Autodesk Inventor part; units mm, degrees
ref_plane "РабПлоскость1" through (0, 0, 80) normal (0, 0, 1) x (1, 0, 0)
ref_plane "YZ Plane" through (0, 0, 0) normal (1, 0, 0) x (0, 1, 0)
ref_plane "XZ Plane" through (0, 0, 0) normal (0, 1, 0) x (-1, 0, 0)
sketch "Эскиз1" plane through (0, 0, 0) normal (0, 0, 1) x (1, 0, 0)
  point P0 (0, 0)
sketch "Эскиз2" plane through (0, 0, 0) normal (0, 0, 1) x (1, 0, 0)
  line L0 (0, 42.5) -> (42.5, 0)
  line L1 (42.5, 0) -> (0, -42.5)
  line L2 (0, -42.5) -> (-42.5, 0)
  line L3 (-42.5, 0) -> (0, 42.5)
  point P0 (0, 0)
  point P1 (0, 0)
  dimension "d0" = 85
sketch "Эскиз3" plane through (0, 0, 0) normal (0, 0, 1) x (1, 0, 0)
  point P0 (0, 0)
ref_plane "РабПлоскость1" through (0, 0, 80) normal (0, 0, 1) x (1, 0, 0)
sketch "Эскиз4" plane through (0, 0, 80) normal (0, 0, 1) x (1, 0, 0)
  point P0 (0, 0)
loft "Лофт1" add profiles "Эскиз2" section 2 point at (0, 0, 80)
sketch "Эскиз5" plane through (0, 0, 0) normal (0, 1, 0) x (-1, 0, 0)
  line L0 (0, 8.7868) -> (-21.2132, 30)
  line L1 (-21.2132, 30) -> (0, 51.2132)
  line L2 (0, 51.2132) -> (21.2132, 30)
  line L3 (21.2132, 30) -> (0, 8.7868)
  line L4 (0, 0) -> (42.5, 0)
  point P0 (0, 30)
  dimension "d6" = 30
  dimension "d7" = 30
extrude "Выдавливание1" cut sketch "Эскиз5" along normal through all both and the other way through all
properties part number "Пирамида"
Could you check a few things on this model? Use its own coordinates, in mm. A direction names the side the tool comes from. Coordinates: 2 decimals unless noted, no trailing zeros. Write each loop counter-clockwise with the first axis right and the second up, starting at its lowest first coordinate (ties: lowest second). Pieces come first, ordered by that corner, then holes. Notation, with made-up numbers: (65, 59) -> (73, 59) arc R26 ccw to (73, 84) -> close; hole circle Ø11 at (75, 32.25). An arc over 180 degrees is marked (long way). Write item = value, one per line. Start each with the question number.
(1) I want a section at C-C (z = 17). Please give me the cut outline in (x, y), plus the area to 3 significant figures.
(2) I want a section at A-A (y = 11). Please give me the cut outline in (x, z).
(3) I want a section at B-B (x = -16). Please give me the cut outline in (y, z).
(4) I need wall thicknesses on line 1 (X direction, y = 15.5, z = 12.5); line 2 (Z direction, x = -7, y = 10.5); line 3 (Z direction, x = 27.5, y = 4.5). Which ranges of each line are inside material? Lowest first, please. Write a range as [from, to].
(5) Which directions (+Z, -Z, +X, -X, +Y, -Y) give clear straight access to the entire face, cutting with the end or side of a thin tool? Please do faces 5 (the face through (-14.9, 15.5, 22.78)), 6 (the face through (-8.398, -0.53, 17.185)).
(6) We'd pull the mould along X, two halves only. Please class faces 1 (the face through (-15.5, -14.9, 22.78)), 2 (the face through (15.5, 14.9, 22.78)), 3 (the face through (1, 1, 0)), 4 (the face through (-8.101, -0.214, 43.112)): released by +X, released by -X, zero draft, split by the parting line, or undercut.
(7) I want a section at D-D (x = 2). Please give me the cut outline in (y, z), plus the area to 3 significant figures.
(8) Will these pins go through, and if not, where does the flat tip stop? pin 1 (12 mm diameter, centred on x = 17, z = 17.5, fed in from +Y); pin 2 (12 mm diameter, centred on x = 13.5, z = 65.5, fed in from +Y); pin 3 (2 mm diameter, centred on x = 15, z = 13, fed in from -Y).
Result set:
q1.outline = (-33.47, 0) -> (-8.21, -25.26) -> (-8.21, 25.26) -> close; (8.21, -25.26) -> (33.47, 0) -> (8.21, 25.26) -> close
q1.area = 1,280 mm2
q2.outline = (-31.5, 0) -> (31.5, 0) -> (17.52, 26.31) -> (0, 8.79) -> (-17.52, 26.31) -> close; (-9.16, 42.05) -> (0, 51.21) -> (9.16, 42.05) -> (0, 59.29) -> close
q3.outline = (-26.5, 0) -> (26.5, 0) -> (13.33, 24.79) -> (-13.33, 24.79) -> close; (-7.79, 35.21) -> (7.79, 35.21) -> (0, 49.88) -> close
q4.line_1 = [-20.36, -3.71], [3.71, 20.36]
q4.line_2 = [0, 15.79], [44.21, 47.06]
q4.line_3 = [0, 19.76]
q5.face_5 = +Z, -X, +Y
q5.face_6 = +Y, -Y
q6.face_1 = released by -X
q6.face_2 = released by +X
q6.face_3 = zero draft
q6.face_4 = undercut
q7.outline = (-40.5, 0) -> (40.5, 0) -> (34.77, 10.79) -> (-34.77, 10.79) -> close; (-14.36, 49.21) -> (14.36, 49.21) -> (0, 76.24) -> close
q7.area = 1,200 mm2
q8.pin_1 = 23
q8.pin_2 = 1
q8.pin_3 = -21.73
